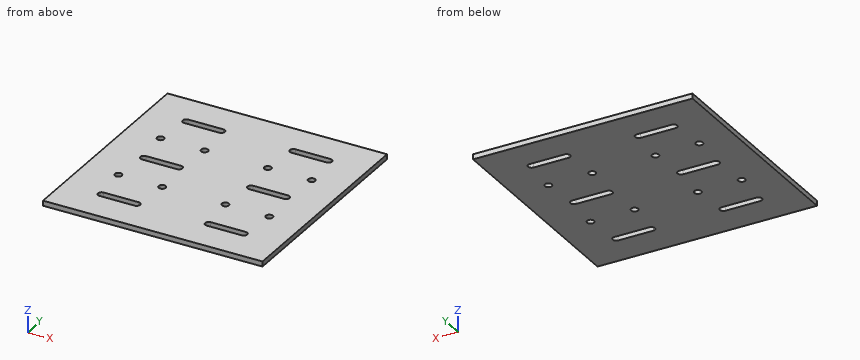
from build123d import *

# Parameters (mm, degrees)
SKETCH_1_W          = 250
SKETCH_1_H          = 250
EXTRUDE_1_DEPTH     = 5.8
CUT_EXTRUDE_1_REACH = 355.601
SKETCH_2_R          = 4


with BuildPart() as part:
    # Эскиз1 → Бобышка-Вытянуть1 (new body)
    with BuildSketch(Plane.XY):
        with Locations((125, 125)):
            Rectangle(SKETCH_1_W, SKETCH_1_H)
        with BuildLine():
            Line((44, 214), (84, 214))
            ThreePointArc((84, 214), (88, 210), (84, 206))
            Line((84, 206), (44, 206))
            ThreePointArc((44, 206), (40, 210), (44, 214))
        make_face(mode=Mode.SUBTRACT)
        with BuildLine():
            Line((166, 214), (206, 214))
            ThreePointArc((206, 214), (210, 210), (206, 206))
            Line((206, 206), (166, 206))
            ThreePointArc((166, 206), (162, 210), (166, 214))
        make_face(mode=Mode.SUBTRACT)
        with BuildLine():
            Line((166, 129), (206, 129))
            ThreePointArc((206, 129), (210, 125), (206, 121))
            Line((206, 121), (166, 121))
            ThreePointArc((166, 121), (162, 125), (166, 129))
        make_face(mode=Mode.SUBTRACT)
        with BuildLine():
            Line((166, 44), (206, 44))
            ThreePointArc((206, 44), (210, 40), (206, 36))
            Line((206, 36), (166, 36))
            ThreePointArc((166, 36), (162, 40), (166, 44))
        make_face(mode=Mode.SUBTRACT)
        with BuildLine():
            Line((44, 129), (84, 129))
            ThreePointArc((84, 129), (88, 125), (84, 121))
            Line((84, 121), (44, 121))
            ThreePointArc((44, 121), (40, 125), (44, 129))
        make_face(mode=Mode.SUBTRACT)
        with BuildLine():
            Line((44, 44), (84, 44))
            ThreePointArc((84, 44), (88, 40), (84, 36))
            Line((84, 36), (44, 36))
            ThreePointArc((44, 36), (40, 40), (44, 44))
        make_face(mode=Mode.SUBTRACT)
    extrude(amount=EXTRUDE_1_DEPTH)

    # Эскиз2 → Вырез-Вытянуть1 (cut, up to next)
    with BuildSketch(Plane.XY.offset(5.8), mode=Mode.PRIVATE) as cut_extrude_1_sk1:
        with Locations((39, 167.5)):
            Circle(SKETCH_2_R)
    cut_extrude_1_tool1 = extrude(cut_extrude_1_sk1.sketch, amount=-CUT_EXTRUDE_1_REACH, mode=Mode.PRIVATE) & part.part
    # Эскиз2 → Вырез-Вытянуть1 (cut, up to next)
    with BuildSketch(Plane.XY.offset(5.8), mode=Mode.PRIVATE) as cut_extrude_1_sk2:
        with Locations((89, 167.5)):
            Circle(SKETCH_2_R)
    cut_extrude_1_tool2 = extrude(cut_extrude_1_sk2.sketch, amount=-CUT_EXTRUDE_1_REACH, mode=Mode.PRIVATE) & part.part
    # Эскиз2 → Вырез-Вытянуть1 (cut, up to next)
    with BuildSketch(Plane.XY.offset(5.8), mode=Mode.PRIVATE) as cut_extrude_1_sk3:
        with Locations((39, 82.5)):
            Circle(SKETCH_2_R)
    cut_extrude_1_tool3 = extrude(cut_extrude_1_sk3.sketch, amount=-CUT_EXTRUDE_1_REACH, mode=Mode.PRIVATE) & part.part
    # Эскиз2 → Вырез-Вытянуть1 (cut, up to next)
    with BuildSketch(Plane.XY.offset(5.8), mode=Mode.PRIVATE) as cut_extrude_1_sk4:
        with Locations((89, 82.5)):
            Circle(SKETCH_2_R)
    cut_extrude_1_tool4 = extrude(cut_extrude_1_sk4.sketch, amount=-CUT_EXTRUDE_1_REACH, mode=Mode.PRIVATE) & part.part
    # Эскиз2 → Вырез-Вытянуть1 (cut, up to next)
    with BuildSketch(Plane.XY.offset(5.8), mode=Mode.PRIVATE) as cut_extrude_1_sk5:
        with Locations((161, 82.5)):
            Circle(SKETCH_2_R)
    cut_extrude_1_tool5 = extrude(cut_extrude_1_sk5.sketch, amount=-CUT_EXTRUDE_1_REACH, mode=Mode.PRIVATE) & part.part
    # Эскиз2 → Вырез-Вытянуть1 (cut, up to next)
    with BuildSketch(Plane.XY.offset(5.8), mode=Mode.PRIVATE) as cut_extrude_1_sk6:
        with Locations((161, 167.5)):
            Circle(SKETCH_2_R)
    cut_extrude_1_tool6 = extrude(cut_extrude_1_sk6.sketch, amount=-CUT_EXTRUDE_1_REACH, mode=Mode.PRIVATE) & part.part
    # Эскиз2 → Вырез-Вытянуть1 (cut, up to next)
    with BuildSketch(Plane.XY.offset(5.8), mode=Mode.PRIVATE) as cut_extrude_1_sk7:
        with Locations((211, 167.5)):
            Circle(SKETCH_2_R)
    cut_extrude_1_tool7 = extrude(cut_extrude_1_sk7.sketch, amount=-CUT_EXTRUDE_1_REACH, mode=Mode.PRIVATE) & part.part
    # Эскиз2 → Вырез-Вытянуть1 (cut, up to next)
    with BuildSketch(Plane.XY.offset(5.8), mode=Mode.PRIVATE) as cut_extrude_1_sk8:
        with Locations((211, 82.5)):
            Circle(SKETCH_2_R)
    cut_extrude_1_tool8 = extrude(cut_extrude_1_sk8.sketch, amount=-CUT_EXTRUDE_1_REACH, mode=Mode.PRIVATE) & part.part
    add(cut_extrude_1_tool1.solids().sort_by_distance((39, 167.5, 5.8))[0], mode=Mode.SUBTRACT)
    add(cut_extrude_1_tool2.solids().sort_by_distance((89, 167.5, 5.8))[0], mode=Mode.SUBTRACT)
    add(cut_extrude_1_tool3.solids().sort_by_distance((39, 82.5, 5.8))[0], mode=Mode.SUBTRACT)
    add(cut_extrude_1_tool4.solids().sort_by_distance((89, 82.5, 5.8))[0], mode=Mode.SUBTRACT)
    add(cut_extrude_1_tool5.solids().sort_by_distance((161, 82.5, 5.8))[0], mode=Mode.SUBTRACT)
    add(cut_extrude_1_tool6.solids().sort_by_distance((161, 167.5, 5.8))[0], mode=Mode.SUBTRACT)
    add(cut_extrude_1_tool7.solids().sort_by_distance((211, 167.5, 5.8))[0], mode=Mode.SUBTRACT)
    add(cut_extrude_1_tool8.solids().sort_by_distance((211, 82.5, 5.8))[0], mode=Mode.SUBTRACT)


solid = part.part
Build history of the part. All positions in model axes, mm. Give positions to 0.01 mm unless a question says otherwise; leave off trailing zeros. Loops run counter-clockwise (first coordinate to the right, second up) from the corner with the lowest first, then second, coordinate; pieces in that order, holes last. Notation, with made-up numbers: (58, -29) -> (78, -29) arc R5 cw to (78, -23) -> close; hole circle Ø8 at (57, -27.5). An arc over 180 degrees is marked (long way). Answer in a Markdown table with one row per item.
Item 1: Slice it at C-C on y = 126. Write the cut outline in (x, z), plus the area to 3 significant figures.
Findings below:
| item | result |
|---|---|
| outline | (0, 0) -> (40.13, 0) -> (40.13, 5.8) -> (0, 5.8) -> close; (87.87, 0) -> (162.13, 0) -> (162.13, 5.8) -> (87.87, 5.8) -> close; (209.87, 0) -> (250, 0) -> (250, 5.8) -> (209.87, 5.8) -> close |
| area | 896 mm² |
Item 2: Slice it at B-B on z = 4. Give the number of separate pieces and of enclosed holes in the cut face, plus the area to 3 significant figures.
Findings below:
| item | result |
|---|---|
| separate pieces | 1 |
| enclosed holes | 14 |
| area | 59,900 mm² |
Item 3: Slice it at A-A on y = 210. Write the cut outline in (x, z), plus the area to 3 significant figures.
Findings below:
| item | result |
|---|---|
| outline | (0, 0) -> (40, 0) -> (40, 5.8) -> (0, 5.8) -> close; (88, 0) -> (162, 0) -> (162, 5.8) -> (88, 5.8) -> close; (210, 0) -> (250, 0) -> (250, 5.8) -> (210, 5.8) -> close |
| area | 893 mm² |
Item 4: Flat gauge pin, fed straight in: P1, Ø6.5, axis at x = 39, y = 167.5, coming from the +Z side. Where does the tip first touch, or does it go through?
Findings below:
| item | result |
|---|---|
| P1 | passes through |
Item 5: Probe line 1 along Y through (x, z) = (211, 1.6); line 2 along Y through (x, z) = (197, 0.2); line 3 along X through (y, z) = (79, 3.25). List the from-to ranges inside material, lowest first. Write a range as [from, to].
Findings below:
| item | result |
|---|---|
| line 1 | y = [0, 78.5], [86.5, 163.5], [171.5, 250] |
| line 2 | y = [0, 36], [44, 121], [129, 206], [214, 250] |
| line 3 | x = [0, 37.06], [40.94, 87.06], [90.94, 159.06], [162.94, 209.06], [212.94, 250] |
